Build history of the part. All positions in model axes, mm. Face numbers are marked on the shaded views. A direction names the side the tool comes from. Round coordinates to 2 decimals unless told otherwise and drop trailing zeros. Write each loop counter-clockwise with the first axis right and the second up, starting at its lowest first coordinate (ties: lowest second). Pieces come first, ordered by that corner, then holes. Notation, with made-up numbers: M 88,66 L 94,66 A17 cw 94,81 Z; hole C -29,67 d7. An arc over 180 degrees is marked long. Write item = value, one per line.
from build123d import *

# Parameters (mm, degrees)
THREADS_SKETCH_W  = 2.5
THREADS_SKETCH_H  = 4
THREADS_CHAM_SIZE = 0.25
NUT_DEPTH         = 2.7
GASKET_SKETCH_R   = 3.5
GASKET_DEPTH      = 0.5
STEM_SKETCH_R     = 1.15
STEM_DEPTH        = 5.3
TOP_START         = 0.3
TOP_FLAT_SKETCH_R = 3.5
TOP_FLAT_DEPTH    = 0.3
PORT_SKETCH_R     = 0.9
PORT_DEPTH        = 14.137097599


with BuildPart() as part:
    # Threads_Sketch → Threads (revolve)
    with BuildSketch(Plane.XY, mode=Mode.PRIVATE) as threads_sk:
        with Locations((-1.25, 2)):
            Rectangle(THREADS_SKETCH_W, THREADS_SKETCH_H)
    revolve(threads_sk.sketch.rotate(Axis((0, 0, 0), (0, 1, 0)), 270), axis=Axis((0, 0, 0), (0, 1, 0)))

    # Threads Cham
    threads_cham_edges = [part.edges().sort_by_distance(p)[0] for p in [
        (0, 0, 2.5),
    ]]
    chamfer(threads_cham_edges, length=THREADS_CHAM_SIZE)

    # Nut_Sketch → Nut (add)
    with BuildSketch(Plane(origin=(0, 4, 0), x_dir=(-1, 0, 0), z_dir=(0, 1, 0))):
        Polygon((-4.041451884, 0), (-2.020725942, -3.5), (2.020725942, -3.5), (4.041451884, 0), (2.020725942, 3.5), (-2.020725942, 3.5), align=None)
    extrude(amount=NUT_DEPTH)

    # Nut Cham_Sketch → Nut Cham (revolve, cut)
    with BuildSketch(Plane.XY, mode=Mode.PRIVATE) as nut_cham_sk:
        Polygon((-4.041451884, 4.312607391), (-4.041451884, 4), (-3.5, 4), align=None)
        Polygon((-3.5, 6.7), (-4.041451884, 6.387392609), (-4.041451884, 6.7), align=None)
    revolve(nut_cham_sk.sketch.rotate(Axis((0, 0, 0), (0, 1, 0)), 90), axis=Axis((0, 0, 0), (0, 1, 0)), mode=Mode.SUBTRACT)

    # Gasket_Sketch → Gasket (add)
    with BuildSketch(Plane.XZ.offset(-4)):
        with Locations(Location((0, 0, 0), (0, 0, 270))):
            Circle(GASKET_SKETCH_R)
    extrude(amount=GASKET_DEPTH)

    # Stem_Sketch → Stem (add)
    with BuildSketch(Plane(origin=(0, 6.7, 0), x_dir=(-1, 0, 0), z_dir=(0, 1, 0))):
        with Locations(Location((0, 0, 0), (0, 0, 90))):
            Circle(STEM_SKETCH_R)
    extrude(amount=STEM_DEPTH)

    # Top Flat_Sketch → Top Flat (add)
    with BuildSketch(Plane(origin=(0, 6.7, 0), x_dir=(-1, 0, 0), z_dir=(0, 1, 0)).offset(TOP_START)):
        with Locations(Location((0, 0, 0), (0, 0, 270))):
            Circle(TOP_FLAT_SKETCH_R)
    extrude(amount=-TOP_FLAT_DEPTH)

    # Outside Barb_Sketch → Outside Barb (revolve)
    with BuildSketch(Plane.XY, mode=Mode.PRIVATE) as outside_barb_sk:
        Polygon((0, 11), (-1.15, 11), (-1.4, 10.5), (-1.4, 10), (0, 10), align=None)
    revolve(outside_barb_sk.sketch.rotate(Axis((0, 0, 0), (0, 1, 0)), 90), axis=Axis((0, 0, 0), (0, 1, 0)))

    # Inside Barb 2_Sketch → Inside Barb 2 (revolve)
    with BuildSketch(Plane.XY, mode=Mode.PRIVATE) as inside_barb_2_sk:
        Polygon((0, 8.5), (-1.15, 8.5), (-1.4, 8.2), (-1.4, 6.7), (0, 6.7), align=None)
    revolve(inside_barb_2_sk.sketch.rotate(Axis((0, 0, 0), (0, 1, 0)), 270), axis=Axis((0, 0, 0), (0, 1, 0)))

    # Port_Sketch → Port (cut, through all)
    with BuildSketch(Plane(origin=(0, 0, 0), x_dir=(1, 0, 0), z_dir=(0, 1, 0))):
        with Locations(Location((0, 0, 0), (0, 0, 270))):
            Circle(PORT_SKETCH_R)
    extrude(amount=PORT_DEPTH, mode=Mode.SUBTRACT)


solid = part.part
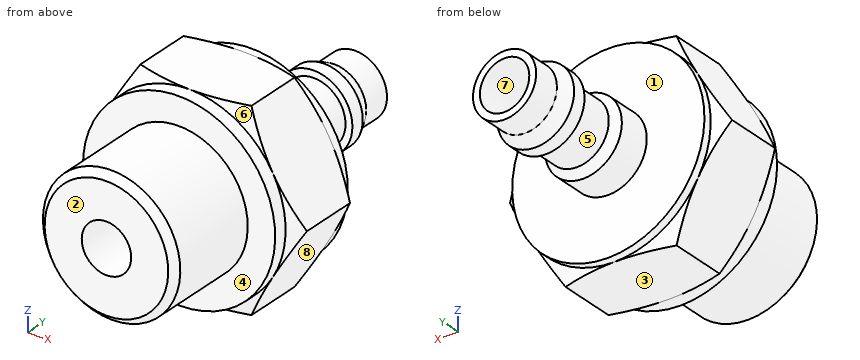
1. Band-saw the part on A-A (y = 7.5). List the corners of the cut face in (x, z).
Responses:
outline = C 0,0 d2.8; hole C 0,0 d1.8
2. Mould opens along Z. For the marked faces 6, 7 and 8 say: pulls with the +Z half, pulls with the -Z half, needs draft (parallel to the pull), parting line crosses it, or undercut.
Responses:
face_6 = pulls with the +Z half
face_7 = undercut
face_8 = pulls with the -Z half
3. Tool access for the marked faces 1, 2, 3, 4 and 5: list every direction of +Z, -Z, +X, -X, +Y, -Y with a clear straight run to the whole face (end or side of a thin tool).
Responses:
face_1 = +Y
face_2 = +Z, -Z, +X, -X, -Y
face_3 = -Z, +X, -X, +Y, -Y
face_4 = -Y
face_5 = none
4. Flat gauge pin, fed straight in: pin 1 (1.5 mm diameter, centred on x = -1.5, z = 2.5, fed in from +Y). Where does the tip first touch, or does it go through?
Responses:
pin_1 = 7
5. Band-saw the part on B-B (y = 2.5). List the corners of the cut face in (x, z), plus the area to 3 significant figures.
Responses:
outline = C 0,0 d5; hole C 0,0 d1.8
area = 17.1 mm²
6. Probe probe 1 along Z at (x, y) = (0, 8.75); probe 2 along X at (y, z) = (7.75, 0). List the from-to ranges inside material, lowest first.
Responses:
probe_1 = -1.15 to -0.9, 0.9 to 1.15
probe_2 = -1.4 to -0.9, 0.9 to 1.4
